Geometry: final body of the model. Coordinates: model frame, mm. Face numbers are marked on the shaded views. A direction names the side the tool comes from. Coordinates: 2 decimals unless noted, no trailing zeros. Order: outer loops, then holes, each group sorted by start corner. A loop starts at its lowest first (then second) coordinate and runs counter-clockwise, first axis right, second up. Notation, with made-up numbers: (-33, 25.5) - (-5, 25.5) arc R37 ccw to (-5, 62.5) - close; hole circle Ø3 at (-4, 4). An arc over 180 degrees is marked (long way). Use one line per item in the form item = value. Start each with the question number.
```python
from build123d import *

# Parameters (mm, degrees)
F0_W      = 50
F0_H      = 40
F1_DEPTH  = 10
F2_R      = 13.825
F3_DEPTH  = 9
F4_R      = 13.5
F5_DEPTH  = 1
F6_W      = 4.25
F6_H      = 8
F7_DEPTH  = 17.515289916
F9_DEPTH  = 12
F10_R     = 5.08
F11_R     = 5.08
F13_DEPTH = 10
F15_DEPTH = 10
F17_DEPTH = 10


with BuildPart() as f1:
    # F0 (on Top) → F1 (new body)
    with BuildSketch(Plane.XY):
        Rectangle(F0_W, F0_H)
    extrude(amount=F1_DEPTH)

    # F2 (on face) → F3 (cut)
    with BuildSketch(Plane(origin=(0, 0, 0), x_dir=(1, 0, 0), z_dir=(0, 0, -1))):
        with Locations((6.175, 0)):
            Circle(F2_R)
    extrude(amount=-F3_DEPTH, mode=Mode.SUBTRACT)

    # F4 (on face) → F5 (cut, through all)
    with BuildSketch(Plane.XY.offset(10)):
        with Locations((6.175, 0)):
            Circle(F4_R)
    extrude(amount=-F5_DEPTH, mode=Mode.SUBTRACT)

    # F6 (on face) → F7 (cut, through all)
    with BuildSketch(Plane(origin=(-25, 0, 0), x_dir=(0, -1, 0), z_dir=(-1, 0, 0))):
        with Locations((0, 4)):
            Rectangle(F6_W, F6_H)
    extrude(amount=-F7_DEPTH, mode=Mode.SUBTRACT)

    # F8 (on face) → F9 (join)
    with BuildSketch(Plane(origin=(-25, 0, 0), x_dir=(0, -1, 0), z_dir=(-1, 0, 0))):
        Polygon((10, 10), (-20, 10), (50.7106781187, -60.7106781187), (65.7106781187, -45.7106781187), align=None)
    extrude(amount=-F9_DEPTH)

    # F10
    f10_edges = [f1.edges().sort_by_distance(p)[0] for p in [
        (25, -20, 5),
        (-25, -20, 5),
        (-25, 20, 5),
        (25, 20, 5),
    ]]
    fillet(f10_edges, radius=F10_R)

    # F11
    f11_edges = [f1.edges().sort_by_distance(p)[0] for p in [
        (-25, -42.855339, -22.855339),
        (-25, -20.355339, -30.355339),
    ]]
    fillet(f11_edges, radius=F11_R)

    # F12 (on face) → F13 (cut)
    with BuildSketch(Plane.YZ.offset(-13)):
        Polygon((2.125, 8), (-2.125, 8), (-2.125, 0), (-56.7731781187, -54.6481781187), (-54.6481781187, -56.7731781187), (2.125, 0), align=None)
    extrude(amount=-F13_DEPTH, mode=Mode.SUBTRACT)

    # F14 (on face) → F15 (join, through all)
    with BuildSketch(Plane.YZ.offset(-13)):
        Polygon((-1.8421572875, -0.2828427125), (-2.125, 0), (-2.8321067812, -0.7071067812), (-2.5492640687, -0.9899494937), align=None)
        Polygon((-16.2671356237, -14.1421356237), (-16.9742424049, -14.8492424049), (-16.6913996924, -15.1320851174), (-15.9842929113, -14.4249783362), align=None)
        Polygon((-30.4092712475, -28.2842712475), (-31.1163780286, -28.9913780286), (-30.8335353162, -29.2742207411), (-30.126428535, -28.5671139599), align=None)
        Polygon((-44.5514068712, -42.4264068712), (-45.2585136524, -43.1335136524), (-44.9756709399, -43.4163563649), (-44.2685641587, -42.7092495837), align=None)
    extrude(amount=-F15_DEPTH)

    # F16 (on face) → F17 (join, through all)
    with BuildSketch(Plane.YZ.offset(-13)):
        Polygon((-8.4852813742, -10.6102813742), (-7.7781745931, -9.9031745931), (-8.0610173055, -9.6203318806), (-8.7681240867, -10.3274386618), align=None)
        Polygon((-22.9102597104, -24.4695742855), (-22.627416998, -24.752416998), (-21.9203102168, -24.0453102168), (-22.2031529293, -23.7624675043), align=None)
        Polygon((-37.0523953342, -38.6117099092), (-36.7695526217, -38.8945526217), (-36.0624458405, -38.1874458405), (-36.345288553, -37.904603128), align=None)
        Polygon((-51.1945309579, -52.753845533), (-50.9116882454, -53.0366882454), (-50.2045814642, -52.3295814642), (-50.4874241767, -52.0467387518), align=None)
    extrude(amount=-F17_DEPTH)


solid = f1.part
```
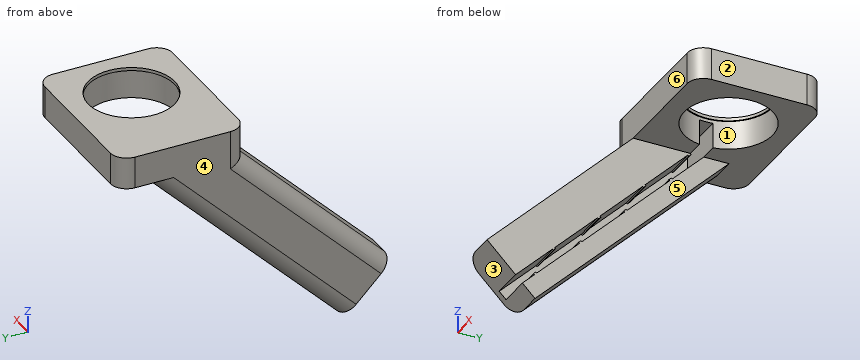
(1) Draft query along X for the marked faces 1, 2 and 3. Return one class per face: released by +X, released by -X, zero draft, split by the parting line, or undercut.
(2) Cut plane B-B on y = 12. Return the cut outline in (x, z), plus the area to 3 significant figures.
(3) Material intervals for L1, parallel to X at y = 0, z = 7.25; L2, parallel to Y at x = -13.5, z = 2.5 (3 decimals); L3, parallel to X at y = -21, z = -27, sorted ascending. Write a range as from..to.
(4) Cut plane A-A on x = 2. Return the cut outline in (y, z), plus the area to 3 significant figures.
(5) Cut plane C-C on x = 22. Return the cut outline in (y, z).
(6) Contact query for flat-ended pins moving along their axis: pin 1 Ø4 at (x, z) = (-12, 5) entering from -Y; pin 2 Ø1 at (y, z) = (-41.5, -35) entering from +X; pin 3 Ø5 at (y, z) = (10, -1) entering from +X; pin 4 Ø3.5 at (x, y) = (-13, -0.5) entering from -Z. Output: stop coordinate, or through.
(7) Set-up query: the marked faces 4, 5 and 6. Return all of +Z, -Z, +X, -X, +Y, -Y with unobstructed straight access to the full face (end or side cutting, diameter ignored); none if empty.
Check sheet entries:
q1.face_1 = undercut
q1.face_2 = released by +X
q1.face_3 = zero draft
q2.outline = (-25, 0) - (-0.69, 0) - (-0.69, 9) - (-0.01, 9) - (-0.01, 10) - (-25, 10) - close; (12.36, 9) - (13.04, 9) - (13.04, 0) - (25, 0) - (25, 10) - (12.36, 10) - close
q2.area = 364 mm^2
q3.L1 = -25..-23, 20..25
q3.L2 = -20..-2.125, 2.125..20
q3.L3 = -24.47..-13
q4.outline = (-20, 0) - (-13.18, 0) - (-13.18, 9) - (-12.84, 9) - (-12.84, 10) - (-20, 10) - close; (12.84, 9) - (13.18, 9) - (13.18, 0) - (20, 0) - (20, 10) - (12.84, 10) - close
q4.area = 137 mm^2
q5.outline = (-19.55, 0) - (19.55, 0) - (19.55, 10) - (-19.55, 10) - close
q6.pin_1 = -20
q6.pin_2 = -13
q6.pin_3 = 25
q6.pin_4 = -12.25
q7.face_4 = +Z, -Z, -X, +Y, -Y
q7.face_5 = -Z, +X, +Y, -Y
q7.face_6 = +Z, +X, -X, -Y
